Work out the finished part from the listing and answer in its coordinate system (mm). A direction names the side the tool comes from. Give positions to 0.01 mm unless a question says otherwise; leave off trailing zeros. Loops run counter-clockwise (first coordinate to the right, second up) from the corner with the lowest first, then second, coordinate; pieces in that order, holes last. Notation, with made-up numbers: M 5,70.25 L 40,70.25 A35 cw 40,108.25 Z; hole C 17.5,1 d3. An arc over 180 degrees is marked long. Answer in a Markdown table with one row per item. Add a question column.
from build123d import *
from build123d.topology import SkipClean

# Parameters (mm, degrees)
SKETCH_1_R           = 17
SKETCH_1_R_2         = 6.5
EXTRUDE_2_DEPTH      = 35
SKETCH_3_W           = 33.795275063
SKETCH_3_H           = 34.72803434
SKETCH_3_R           = 13
EXTRUDE_7_DEPTH      = 45
SKETCH_4_R           = 6.5
CUT_EXTRUDE_1_DEPTH  = 60.489495005
SKETCH_12_R          = 2
CUT_EXTRUDE_11_DEPTH = 45
SKETCH_15_R          = 2
CUT_EXTRUDE_12_DEPTH = 45
FILLET_4_R           = 10
SKETCH_20_R          = 13
CUT_EXTRUDE_18_DEPTH = 31
EXTRUDE_START        = 1
SKETCH_25_R          = 13
EXTRUDE_10_DEPTH     = 1


with BuildPart() as part:
    # Эскиз1 → Бобышка-Вытянуть2 (new body)
    with BuildSketch(Plane.XY):
        Circle(SKETCH_1_R)
        Circle(SKETCH_1_R_2, mode=Mode.SUBTRACT)
    extrude(amount=EXTRUDE_2_DEPTH)

    # Эскиз3 → Бобышка-Вытянуть7 (add)
    with BuildSketch(Plane(origin=(0, 45, 0), x_dir=(1, 0, 0), z_dir=(0, 1, 0))):
        with Locations((0.102362468, -17.511098906)):
            Rectangle(SKETCH_3_W, SKETCH_3_H)
        with Locations(Location((0, -17.5, 0), (0, 0, 270))):
            Circle(SKETCH_3_R, mode=Mode.SUBTRACT)
    extrude(amount=-EXTRUDE_7_DEPTH)

    # Эскиз4 → Вырез-Вытянуть1 (cut, through all)
    with BuildSketch(Plane(origin=(0, 0, 0), x_dir=(-1, 0, 0), z_dir=(0, 0, -1))):
        with Locations(Location((0, 0, 0), (0, 0, 180))):
            Circle(SKETCH_4_R)
    extrude(amount=-CUT_EXTRUDE_1_DEPTH, mode=Mode.SUBTRACT)

    # Эскиз12 → Вырез-Вытянуть11 (cut)
    with BuildSketch(Plane(origin=(0, 0, 0), x_dir=(-1, 0, 0), z_dir=(0, 0, -1))):
        with Locations((0, 23)):
            Circle(SKETCH_12_R)
    extrude(amount=-CUT_EXTRUDE_11_DEPTH, mode=Mode.SUBTRACT)

    # Эскиз15 → Вырез-Вытянуть12 (cut)
    with BuildSketch(Plane.ZY.offset(16.795275063)):
        with Locations((17.5, 33)):
            Circle(SKETCH_15_R)
    extrude(amount=-CUT_EXTRUDE_12_DEPTH, mode=Mode.SUBTRACT)

    # Скругление4
    # the kernel refuses this fillet: 10 mm, written as the material it takes off along each edge
    with BuildSketch(Plane(origin=(-16.795275063, 70, 34.875116076), x_dir=(1, 0, 0), z_dir=(0, -1, 0))) as fillet_4_piece_1_section:
        with BuildLine():
            CenterArc((FILLET_4_R, -FILLET_4_R), FILLET_4_R, 90, 90)
            Line((0, -FILLET_4_R), (0, 0))
            Line((0, 0), (FILLET_4_R, 0))
        make_face()
    fillet_4_piece_1 = extrude(amount=92.369651061, mode=Mode.PRIVATE)
    fillet_4_piece_1 = fillet_4_piece_1 - Plane(origin=(0, 0, 32.54483178), x_dir=(1, 0, 0), z_dir=(0, 0, -1)) * Cylinder(17, 225, mode=Mode.PRIVATE)
    add(fillet_4_piece_1, mode=Mode.SUBTRACT)
    with BuildSketch(Plane(origin=(17, 70, 0.147081736), x_dir=(0, 0, 1), z_dir=(0, -1, 0))) as fillet_4_piece_2_section:
        with BuildLine():
            CenterArc((FILLET_4_R, FILLET_4_R), FILLET_4_R, 180, 90)
            Line((0, FILLET_4_R), (0, 0))
            Line((0, 0), (FILLET_4_R, 0))
        make_face()
    fillet_4_piece_2 = extrude(amount=95, mode=Mode.PRIVATE)
    fillet_4_piece_2 = fillet_4_piece_2 - Plane(origin=(0, 0, 2.486350956), x_dir=(1, 0, 0), z_dir=(0, 0, -1)) * Cylinder(17, 230, mode=Mode.PRIVATE)
    add(fillet_4_piece_2, mode=Mode.SUBTRACT)
    with BuildSketch(Plane(origin=(17, 70, 34.875116076), x_dir=(0, 0, -1), z_dir=(0, -1, 0))) as fillet_4_piece_3_section:
        with BuildLine():
            CenterArc((FILLET_4_R, -FILLET_4_R), FILLET_4_R, 90, 90)
            Line((0, -FILLET_4_R), (0, 0))
            Line((0, 0), (FILLET_4_R, 0))
        make_face()
    fillet_4_piece_3 = extrude(amount=95, mode=Mode.PRIVATE)
    fillet_4_piece_3 = fillet_4_piece_3 - Plane(origin=(0, 0, 32.535846855), x_dir=(1, 0, 0), z_dir=(0, 0, -1)) * Cylinder(17, 230, mode=Mode.PRIVATE)
    add(fillet_4_piece_3, mode=Mode.SUBTRACT)
    with BuildSketch(Plane(origin=(-16.795275063, 70, 0.147081736), x_dir=(0, 0, 1), z_dir=(0, -1, 0))) as fillet_4_piece_4_section:
        with BuildLine():
            CenterArc((FILLET_4_R, -FILLET_4_R), FILLET_4_R, 90, 90)
            Line((0, -FILLET_4_R), (0, 0))
            Line((0, 0), (FILLET_4_R, 0))
        make_face()
    fillet_4_piece_4 = extrude(amount=92.369651061, mode=Mode.PRIVATE)
    fillet_4_piece_4 = fillet_4_piece_4 - Plane(origin=(0, 0, 2.477367304), x_dir=(1, 0, 0), z_dir=(0, 0, -1)) * Cylinder(17, 225, mode=Mode.PRIVATE)
    add(fillet_4_piece_4, mode=Mode.SUBTRACT)

    # Эскиз20 → Вырез-Вытянуть18 (cut)
    with SkipClean():  # the faces are left unmerged after this step: merging them gives an invalid solid
        with BuildSketch(Plane(origin=(0, 45, 0), x_dir=(1, 0, 0), z_dir=(0, 1, 0))):
            with Locations(Location((0, -17.5, 0), (0, 0, 270))):
                Circle(SKETCH_20_R)
        extrude(amount=-CUT_EXTRUDE_18_DEPTH, mode=Mode.SUBTRACT)

    # Эскиз25 → Бобышка-Вытянуть10 (add)
    with BuildSketch(Plane(origin=(0, 14, 0), x_dir=(1, 0, 0), z_dir=(0, 1, 0)).offset(EXTRUDE_START)):
        with Locations(Location((0, -17.5, 0), (0, 0, 270))):
            Circle(SKETCH_25_R)
    extrude(amount=-EXTRUDE_10_DEPTH)


solid = part.part
(1) Section B-B, the plane y = 33 is taken. Determine the outline of the cut face in (x, z).
(2) Section A-A, the plane x = 0 is taken. Determine the outline of the cut face in (y, z).
(3) Section D-D, the plane z = 27 is taken. Determine the outline of the cut face in (x, y), and give its area (3 significant figures).
(4) Each of these flat-tipped pins is pushed along its axis until it touches: P1, Ø11, axis at x = 3, y = 32.5, coming from the -Z side; P2, Ø7.5, axis at y = 13.5, z = 20.5, coming from the -X side; P3, Ø10, axis at x = -12, z = 30.5, coming from the -Y side. Where does it stop, or does it pass through?
(5) Section C-C, the plane z = 11 is taken. Determine the outline of the cut face in (x, y), and give its area (3 significant figures).
(6) The mould has two halves that part along Y. Classify faces 5 (the face through (11, 45, 10)), 6 (the face through (-13.79, 28.82, 32.02)), 7 (the face through (11.07, 12.9, 17.38)): pulls with the +Y half, pulls with the -Y half, needs draft (parallel to the pull), parting line crosses it, or undercut.
(7) Consider line 1 along Y through (x, z) = (0, 1.75); line 2 along X through (y, z) = (26, 17); line 3 along Y through (x, z) = (0, 9). Determine where each line is inside the solid, lowest interval first. Write a range as from..to.
(8) Which of the six approach directions +Z, -Z, +X, -X, +Y, -Y give full straight-line access (tool end or side, diameter ignored) to faces 1 (the face through (13.993, 27.815, 2.999)), 2 (the face through (13, 12.8, 17.6)), 3 (the face through (-13.94, 28.82, 3.15)), 4 (the face through (0, 15, 17))?
Numbers:
| question | item | result |
|---|---|---|
| 1 | outline | M -16.8,10.15 A10 ccw -6.8,0.15 L 7,0.15 A10 ccw 17,10.15 L 17,15.5 L 12.85,15.5 A13 cw -12.85,15.5 L -16.8,15.5 Z; M -16.8,19.5 L -12.85,19.5 A13 cw 12.85,19.5 L 17,19.5 L 17,24.88 A10 ccw 7,34.88 L -6.8,34.88 A10 ccw -16.8,24.88 Z |
| 2 | outline | M -17,0 L -6.5,0 L -6.5,35 L -17,35 Z; M 6.5,0 L 17,0 L 17,0.15 L 21,0.15 L 21,4.5 L 15,4.5 L 15,30.5 L 21,30.5 L 21,34.88 L 17,34.88 L 17,35 L 6.5,35 Z; M 25,0.15 L 45,0.15 L 45,4.5 L 25,4.5 Z; M 25,30.5 L 45,30.5 L 45,34.88 L 25,34.88 Z |
| 3 | outline | M -16.57,3.81 A17 ccw long 16.77,2.78 L 16.77,45 L 8.87,45 L 8.87,15 L -8.87,15 L -8.87,45 L -16.57,45 Z; hole C 0,0 d13 |
| 3 | area | 1,290 mm² |
| 4 | P1 | stops at z = 0.15 |
| 4 | P2 | stops at x = -16.8 |
| 4 | P3 | stops at y = -15.49 |
| 5 | outline | M -16.8,2.63 A17 ccw long 17,0 L 17,45 L 11.26,45 L 11.26,15 L -11.26,15 L -11.26,45 L -16.8,45 Z; hole M -11.26,12.74 A17 cw -9.64,14 L -11.26,14 Z; hole C 0,0 d13; hole M 9.64,14 A17 cw 11.26,12.74 L 11.26,14 Z |
| 5 | area | 1,160 mm² |
| 6 | face 5 | pulls with the +Y half |
| 6 | face 6 | needs draft |
| 6 | face 7 | undercut |
| 7 | line 1 | y = -17..-6.5, 6.5..21, 25..45 |
| 7 | line 2 | x = -16.8..-12.99, 12.99..17 |
| 7 | line 3 | y = -17..-6.5, 6.5..15 |
| 8 | face 1 | -Z, +X, +Y |
| 8 | face 2 | none |
| 8 | face 3 | -Z, -X, +Y |
| 8 | face 4 | +Y |
